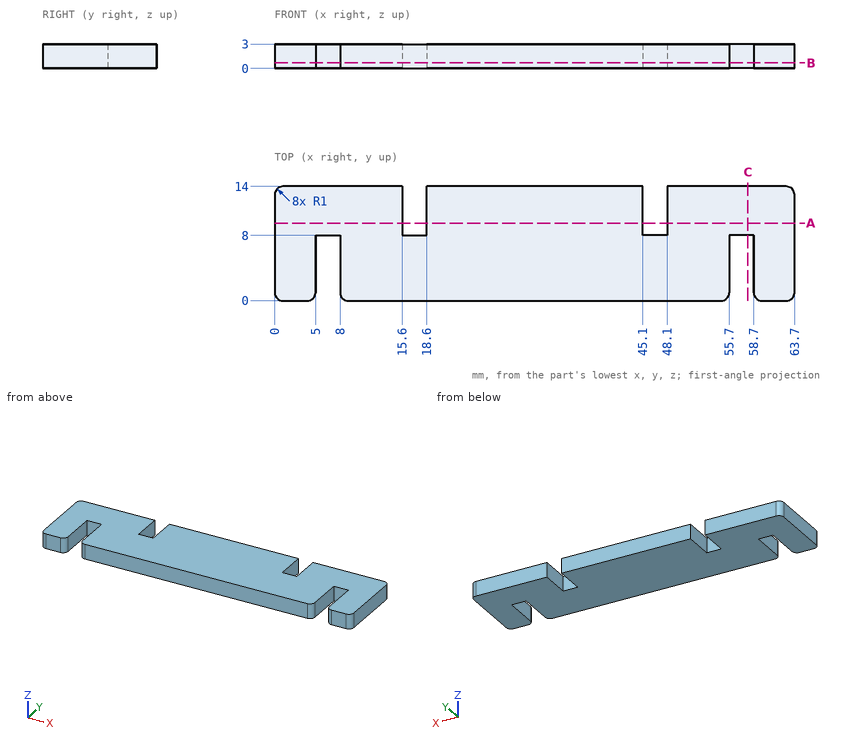
Here's the drawing with two shaded views (mm, measured from the low corner). I have some questions. Give positions to 0.01 mm unless a question says otherwise; leave off trailing zeros. Order: outer loops, then holes, each group sorted by start corner. A loop starts at its lowest first (then second) coordinate and runs counter-clockwise, first axis right, second up. Notation, with made-up numbers: (74, 24.5) -> (122, 24.5) arc R28 ccw to (122, 57.5) -> close; hole circle Ø11 at (61.5, 80). An arc over 180 degrees is marked (long way). One line per item, written item: value. Start each with the question number.
1. Will this pin go through, and if not, where does the flat tip stop? pin 1 Ø0.9 at (x, z) = (6, 1.5) entering from -Y.
2. Imagine slicing it at C-C, the plane x = 58. List the corners of the cut face in (y, z) for me, plus the area to 3 significant figures.
3. Imagine slicing it at B-B, the plane z = 0.7. List the corners of the cut face in (x, y) for me, plus the area to 3 significant figures.
4. Imagine slicing it at A-A, the plane y = 9.5. List the corners of the cut face in (x, z) for me.
5. I need wall thicknesses on probe 1 along X at (y, z) = (6.5, 2); probe 2 along X at (y, z) = (8.25, 2.65); probe 3 along Y at (x, z) = (6, 2.4). Which ranges of each line are inside material? Lowest first, please. Write a range as from..to.
Values follow:
1. pin 1: stops at y = 8
2. outline: (8, 0) -> (14, 0) -> (14, 3) -> (8, 3) -> close
2. area: 18.0 mm2
3. outline: (0, 1) arc R1 ccw to (1, 0) -> (4, 0) arc R1 ccw to (5, 1) -> (5, 8) -> (8, 8) -> (8, 1) arc R1 ccw to (9, 0) -> (54.7, 0) arc R1 ccw to (55.7, 1) -> (55.7, 8) -> (58.7, 8) -> (58.7, 1) arc R1 ccw to (59.7, 0) -> (62.7, 0) arc R1 ccw to (63.7, 1) -> (63.7, 13) arc R1 ccw to (62.7, 14) -> (48.1, 14) -> (48.1, 8) -> (45.1, 8) -> (45.1, 14) -> (18.6, 14) -> (18.6, 8) -> (15.6, 8) -> (15.6, 14) -> (1, 14) arc R1 ccw to (0, 13) -> close
3. area: 806 mm2
4. outline: (0, 0) -> (15.6, 0) -> (15.6, 3) -> (0, 3) -> close; (18.6, 0) -> (45.1, 0) -> (45.1, 3) -> (18.6, 3) -> close; (48.1, 0) -> (63.7, 0) -> (63.7, 3) -> (48.1, 3) -> close
5. probe 1: x = 0..5, 8..55.7, 58.7..63.7
5. probe 2: x = 0..15.6, 18.6..45.1, 48.1..63.7
5. probe 3: y = 8..14
